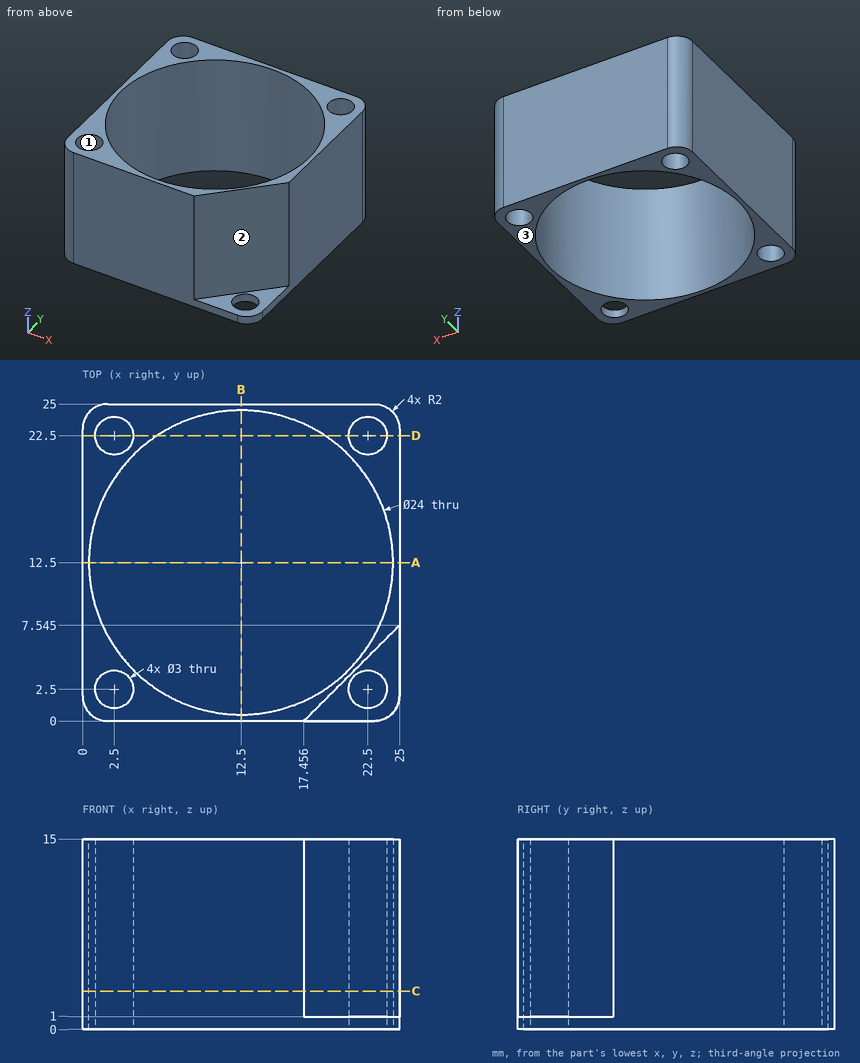
The drawing under review shows one solid part. Ordinate dimensions are in mm from its lowest x, y, z. Coordinates: 2 decimals unless noted, no trailing zeros. Write each loop counter-clockwise with the first axis right and the second up, starting at its lowest first coordinate (ties: lowest second). Pieces come first, ordered by that corner, then holes. Notation, with made-up numbers: M 17,25.25 L 72,25.25 A10 cw 72,41.25 Z; hole C -19.5,-31.5 d6. An arc over 180 degrees is marked long. Answer as a JSON object with one key per item and string values.
Item 1: Add section A-A, the plane y = 12.5. Give the boundary of the cut face in (x, z).
Outcome:
{"outline": "M 0,0 L 0.5,0 L 0.5,15 L 0,15 Z; M 24.5,0 L 25,0 L 25,15 L 24.5,15 Z"}
Item 2: Add section D-D, the plane y = 22.5. Give the boundary of the cut face in (x, z).
Outcome:
{"outline": "M 0,0 L 1,0 L 1,15 L 0,15 Z; M 4,0 L 5.87,0 L 5.87,15 L 4,15 Z; M 19.13,0 L 21,0 L 21,15 L 19.13,15 Z; M 24,0 L 25,0 L 25,15 L 24,15 Z"}
Item 3: Add section C-C, the plane z = 3. Give the boundary of the cut face in (x, y) (1 decimal).
Outcome:
{"outline": "M 0,2 A2 ccw 2,0 L 17.5,0 L 25,7.5 L 25,23 A2 ccw 23,25 L 2,25 A2 ccw 0,23 Z; hole C 12.5,12.5 d24; hole C 2.5,2.5 d3; hole C 2.5,22.5 d3; hole C 22.5,22.5 d3"}
Item 4: Wall thickness on probe 1 along Y at (x, z) = (12.5, 8.5); probe 2 along Y at (x, z) = (22.5, 3.25) (1 decimal); probe 3 along Y at (x, z) = (2.5, 8) (1 decimal): over which ranges is each line inside the solid? List them lowest first.
Outcome:
{"probe 1": "0 to 0.5, 24.5 to 25", "probe 2": "5 to 5.9, 19.1 to 21, 24 to 25", "probe 3": "0 to 1, 4 to 5.9, 19.1 to 21, 24 to 25"}
Item 5: Draft analysis for pull direction X (two halves, no side actions). For the marked faces 1, 2 and 3, state which applies: pulls with the +X half, pulls with the -X half, needs draft (parallel to the pull), parting line crosses it, or undercut.
Outcome:
{"face 1": "undercut", "face 2": "pulls with the +X half", "face 3": "needs draft"}
